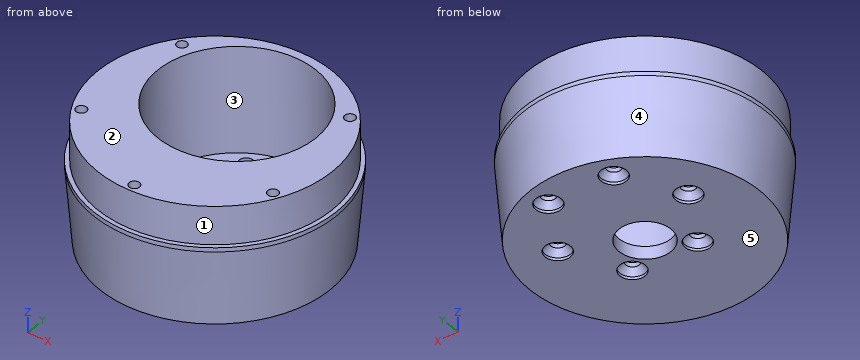
```python
from build123d import *

# Parameters (mm, degrees)
SKETCH1_R              = 28.7
SKETCH1_R_2            = 6.15
SKETCH1_R_3            = 1.65
EXTRUDE_510_DEPTH      = 28
SKETCH2_R              = 18.7
CUT_EXTRUDE_689_DEPTH  = 25
CUT_EXTRUDE_START      = -9
SKETCH4_R              = 28.7
SKETCH4_R_2            = 27.7
CUT_EXTRUDE_844_DEPTH  = 9
SKETCH5_R              = 1.25
SKETCH5_R_2            = 1.2
CUT_EXTRUDE_1374_DEPTH = 10
SKETCH_1_R             = 3
CUT_EXTRUDE_1690_DEPTH = 0.5
CHAMFER_1743_SIZE      = 1.5
CHAMFER_1_SIZE         = 1.5
CHAMFER_1_SIZE2        = 18


with BuildPart() as part:
    # Sketch1 → Extrude 510 (new body)
    with BuildSketch(Plane.XY):
        Circle(SKETCH1_R)
        Circle(SKETCH1_R_2, mode=Mode.SUBTRACT)
        with Locations((15.5, 7)):
            Circle(SKETCH1_R_3, mode=Mode.SUBTRACT)
        with Locations((7.75, -6.423393759)):
            Circle(SKETCH1_R_3, mode=Mode.SUBTRACT)
        with Locations((-7.75, -6.423393759)):
            Circle(SKETCH1_R_3, mode=Mode.SUBTRACT)
        with Locations((-15.5, 7)):
            Circle(SKETCH1_R_3, mode=Mode.SUBTRACT)
        with Locations((-7.75, 20.423393759)):
            Circle(SKETCH1_R_3, mode=Mode.SUBTRACT)
        with Locations((7.75, 20.423393759)):
            Circle(SKETCH1_R_3, mode=Mode.SUBTRACT)
    extrude(amount=EXTRUDE_510_DEPTH)

    # Sketch2 → Cut-Extrude 689 (cut)
    with BuildSketch(Plane.XY.offset(28)):
        with Locations((0, 7)):
            Circle(SKETCH2_R)
    extrude(amount=-CUT_EXTRUDE_689_DEPTH, mode=Mode.SUBTRACT)

    # Sketch4 → Cut-Extrude 844 (cut)
    with BuildSketch(Plane.XY.offset(28).offset(CUT_EXTRUDE_START)):
        Circle(SKETCH4_R)
        Circle(SKETCH4_R_2, mode=Mode.SUBTRACT)
    extrude(amount=CUT_EXTRUDE_844_DEPTH, mode=Mode.SUBTRACT)

    # Sketch5 → Cut-Extrude 1374 (cut)
    with BuildSketch(Plane.XY.offset(28)):
        with Locations((-22.74001983, -12.081142252)):
            Circle(SKETCH5_R)
        with Locations((0, -25.75)):
            Circle(SKETCH5_R)
        with Locations(Location((19.936884337, 16.296721846, 0), (0, 0, 180))):
            Circle(SKETCH5_R)
        with Locations(Location((22.74001983, -12.081142252, 0), (0, 0, 180))):
            Circle(SKETCH5_R)
        with Locations((-19.936884337, 16.296721846)):
            Circle(SKETCH5_R_2)
    extrude(amount=-CUT_EXTRUDE_1374_DEPTH, mode=Mode.SUBTRACT)

    # Эскиз1 → Cut-Extrude 1690 (cut)
    with BuildSketch(Plane(origin=(0, 0, 0), x_dir=(-1, 0, 0), z_dir=(0, 0, -1))):
        with Locations((-7.75, 20.423393759)):
            Circle(SKETCH_1_R)
        with Locations((7.75, 20.423393759)):
            Circle(SKETCH_1_R)
        with Locations((15.5, 7)):
            Circle(SKETCH_1_R)
        with Locations((7.75, -6.423393759)):
            Circle(SKETCH_1_R)
        with Locations((-7.75, -6.423393759)):
            Circle(SKETCH_1_R)
        with Locations((-15.5, 7)):
            Circle(SKETCH_1_R)
    extrude(amount=-CUT_EXTRUDE_1690_DEPTH, mode=Mode.SUBTRACT)

    # Chamfer 1743
    # the kernel refuses this chamfer: 1.5 mm, written as the material it takes off along each edge
    with BuildSketch(Plane(origin=(15.5, 7, 0.5), x_dir=(1, 0, 0), z_dir=(0, 1, 0))) as chamfer_1743_piece_1_section:
        Polygon((1.65 + CHAMFER_1743_SIZE, 0), (1.65, -CHAMFER_1743_SIZE), (1.65, 0), align=None)
    chamfer_1743_piece_1 = revolve(axis=Axis((15.5, 7, 0.5), (0, 0, -1)), mode=Mode.PRIVATE)
    chamfer_1743_piece_1 = chamfer_1743_piece_1 & Plane(origin=(15.5, 7, 1.328305934), x_dir=(-1, 0, 0), z_dir=(0, 0, -1)) * Cylinder(3, 13, mode=Mode.PRIVATE)
    add(chamfer_1743_piece_1, mode=Mode.SUBTRACT)
    with BuildSketch(Plane(origin=(7.75, -6.423393759, 0.5), x_dir=(1, 0, 0), z_dir=(0, 1, 0))) as chamfer_1743_piece_2_section:
        Polygon((1.65 + CHAMFER_1743_SIZE, 0), (1.65, -CHAMFER_1743_SIZE), (1.65, 0), align=None)
    chamfer_1743_piece_2 = revolve(axis=Axis((7.75, -6.423393759, 0.5), (0, 0, -1)), mode=Mode.PRIVATE)
    chamfer_1743_piece_2 = chamfer_1743_piece_2 & Plane(origin=(7.75, -6.423393759, 1.328305934), x_dir=(-1, 0, 0), z_dir=(0, 0, -1)) * Cylinder(3, 13, mode=Mode.PRIVATE)
    add(chamfer_1743_piece_2, mode=Mode.SUBTRACT)
    with BuildSketch(Plane(origin=(-7.75, -6.423393759, 0.5), x_dir=(1, 0, 0), z_dir=(0, 1, 0))) as chamfer_1743_piece_3_section:
        Polygon((1.65 + CHAMFER_1743_SIZE, 0), (1.65, -CHAMFER_1743_SIZE), (1.65, 0), align=None)
    chamfer_1743_piece_3 = revolve(axis=Axis((-7.75, -6.423393759, 0.5), (0, 0, -1)), mode=Mode.PRIVATE)
    chamfer_1743_piece_3 = chamfer_1743_piece_3 & Plane(origin=(-7.75, -6.423393759, 1.328305934), x_dir=(-1, 0, 0), z_dir=(0, 0, -1)) * Cylinder(3, 13, mode=Mode.PRIVATE)
    add(chamfer_1743_piece_3, mode=Mode.SUBTRACT)
    with BuildSketch(Plane(origin=(-15.5, 7, 0.5), x_dir=(1, 0, 0), z_dir=(0, 1, 0))) as chamfer_1743_piece_4_section:
        Polygon((1.65 + CHAMFER_1743_SIZE, 0), (1.65, -CHAMFER_1743_SIZE), (1.65, 0), align=None)
    chamfer_1743_piece_4 = revolve(axis=Axis((-15.5, 7, 0.5), (0, 0, -1)), mode=Mode.PRIVATE)
    chamfer_1743_piece_4 = chamfer_1743_piece_4 & Plane(origin=(-15.5, 7, 1.328305934), x_dir=(-1, 0, 0), z_dir=(0, 0, -1)) * Cylinder(3, 13, mode=Mode.PRIVATE)
    add(chamfer_1743_piece_4, mode=Mode.SUBTRACT)
    with BuildSketch(Plane(origin=(-7.75, 20.423393759, 0.5), x_dir=(1, 0, 0), z_dir=(0, 1, 0))) as chamfer_1743_piece_5_section:
        Polygon((1.65 + CHAMFER_1743_SIZE, 0), (1.65, -CHAMFER_1743_SIZE), (1.65, 0), align=None)
    chamfer_1743_piece_5 = revolve(axis=Axis((-7.75, 20.423393759, 0.5), (0, 0, -1)), mode=Mode.PRIVATE)
    chamfer_1743_piece_5 = chamfer_1743_piece_5 & Plane(origin=(-7.75, 20.423393759, 1.328305934), x_dir=(-1, 0, 0), z_dir=(0, 0, -1)) * Cylinder(3, 13, mode=Mode.PRIVATE)
    add(chamfer_1743_piece_5, mode=Mode.SUBTRACT)
    with BuildSketch(Plane(origin=(7.75, 20.423393759, 0.5), x_dir=(1, 0, 0), z_dir=(0, 1, 0))) as chamfer_1743_piece_6_section:
        Polygon((1.65 + CHAMFER_1743_SIZE, 0), (1.65, -CHAMFER_1743_SIZE), (1.65, 0), align=None)
    chamfer_1743_piece_6 = revolve(axis=Axis((7.75, 20.423393759, 0.5), (0, 0, -1)), mode=Mode.PRIVATE)
    chamfer_1743_piece_6 = chamfer_1743_piece_6 & Plane(origin=(7.75, 20.423393759, 1.328305934), x_dir=(-1, 0, 0), z_dir=(0, 0, -1)) * Cylinder(3, 13, mode=Mode.PRIVATE)
    add(chamfer_1743_piece_6, mode=Mode.SUBTRACT)

    # Фаска1
    chamfer_1_edges = [part.edges().sort_by_distance(p)[0] for p in [
        (-28.7, 0, 0),
    ]]
    chamfer_1_side = [part.faces().sort_by_distance(p)[0] for p in [
        (-27.888241415, 0, 0),
    ]]
    chamfer(chamfer_1_edges, length=CHAMFER_1_SIZE, length2=CHAMFER_1_SIZE2, reference=chamfer_1_side[0])


solid = part.part
```
Geometry: final body of the model. Coordinates: model frame, mm. Face numbers are marked on the shaded views. A direction names the side the tool comes from. Coordinates: 2 decimals unless noted, no trailing zeros. Write each loop counter-clockwise with the first axis right and the second up, starting at its lowest first coordinate (ties: lowest second). Pieces come first, ordered by that corner, then holes. Notation, with made-up numbers: M 78,-19 L 104,-19 A5 cw 104,-13 Z; hole C 47.25,-25 d6. An arc over 180 degrees is marked long. Answer as CSV lines item,"result". Start each with the question number.
Q1. Mould query, pull axis Y, two halves, no side actions, for the marked faces 3, 4 and 5. Classes: released by +Y, released by -Y, zero draft, split by the parting line, or undercut.
Q2. Reachability of the marked faces 1 and 2 from +Z, -Z, +X, -X, +Y, -Y: full face, straight path, thin tool, end or side. Return the list, or none.
Q3. Cut plane A-A on x = 0. Return the cut outline in (y, z), then the cut area to 3 significant figures.
Q4. Pin query (flat end, axial travel): P1, Ø10, axis at y = 16.5, z = 14.5, coming from the -X side; P2, Ø3, axis at x = 15.5, y = 7, coming from the +Z side; P3, Ø5.5, axis at x = -7.75, y = 20.42, coming from the +Z side; P4, Ø1.2, axis at x = -23, y = -12, coming from the +Z side. Return the tip coordinate at first contact, or that it passes through.
Q5. Line query: line 1 (Y direction, x = -7.75, z = 2.3); line 2 (X direction, y = 7, z = 0.15); line 3 (X direction, y = 17, z = 18.25). Output: solid intervals per line, ascending. Write a range as from..to.
Q6. Cut plane B-B on y = 0. Return the cut outline in (x, z).
Q7. Cut plane D-D on z = 16. Return the cut outline in (x, y).
Q8. Cut plane C-C on z = 22.5. Return the cut outline in (x, y), then the cut area to 3 significant figures.
Findings below:
1,face 3,"undercut"
1,face 4,"split by the parting line"
1,face 5,"zero draft"
2,face 1,"+Z"
2,face 2,"+Z, +X, -X, +Y, -Y"
3,outline,"M -28.7,18 L -27.2,0 L -6.15,0 L -6.15,3 L -11.7,3 L -11.7,28 L -24.5,28 L -24.5,18 L -27,18 L -27,28 L -27.7,28 L -27.7,19 L -28.7,19 Z; M 6.15,0 L 27.2,0 L 28.7,18 L 28.7,19 L 27.7,19 L 27.7,28 L 25.7,28 L 25.7,3 L 6.15,3 Z"
3,area,"565 mm2"
4,P1,"stops at x = -26.02"
4,P2,"passes through"
4,P3,"stops at z = 3"
4,P4,"stops at z = 18"
5,line 1,"y = -26.27..-8.07, -4.77..18.77, 22.07..26.27"
5,line 2,"x = -26.3..-18.5, -12.5..12.5, 18.5..26.3"
5,line 3,"x = -23.12..-20.91, -18.96..-15.8, 15.8..18.9, 20.97..23.12"
6,outline,"M -28.7,18 L -27.2,0 L -6.15,0 L -6.15,3 L -17.34,3 L -17.34,28 L -27.7,28 L -27.7,19 L -28.7,19 Z; M 6.15,0 L 27.2,0 L 28.7,18 L 28.7,19 L 27.7,19 L 27.7,28 L 17.34,28 L 17.34,3 L 6.15,3 Z"
7,outline,"C 0,0 d57.07; hole C 0,7 d37.4"
8,outline,"C 0,0 d55.4; hole C -22.74,-12.08 d2.5; hole C -19.94,16.3 d2.4; hole C 0,7 d37.4; hole C 0,-25.75 d2.5; hole C 19.94,16.3 d2.5; hole C 22.74,-12.08 d2.5"
8,area,"1,290 mm2"
